```python
from build123d import *

# Parameters (mm, degrees)
SKETCH1_W           = 190
SKETCH1_H           = 219
BOSS_EXTRUDE1_DEPTH = 2
SKETCH4_W           = 70
SKETCH4_H           = 60
CUT_EXTRUDE1_DEPTH  = 4
SKETCH2_W           = 30
SKETCH2_H           = 2
BOSS_EXTRUDE2_DEPTH = 20
SKETCH3_W           = 190
SKETCH3_H           = 70
BOSS_EXTRUDE3_DEPTH = 72
SKETCH7_R           = 3
SKETCH7_R_2         = 4.5
BOSS_EXTRUDE4_DEPTH = 4
SKETCH8_R           = 3.5
CUT_EXTRUDE3_DEPTH  = 4
SKETCH9_R           = 2
BOSS_EXTRUDE5_DEPTH = 2
SKETCH10_R          = 0.95
CUT_EXTRUDE4_DEPTH  = 2
SKETCH11_R          = 1.875
SKETCH11_R_2        = 4.75
CUT_EXTRUDE5_DEPTH  = 4
SKETCH12_R          = 4.5
BOSS_EXTRUDE6_DEPTH = 72
SKETCH13_R          = 3.5
CUT_EXTRUDE6_DEPTH  = 4.5
FILLET1_START       = 2
FILLET1_DEPTH       = 73
FILLET1_START_2     = 22
FILLET1_2_DEPTH     = 53
FILLET1_START_3     = -1
FILLET1_3_DEPTH     = 23
SKETCH14_W          = 18
SKETCH14_H          = 15
CUT_EXTRUDE7_DEPTH  = 5
SKETCH15_R          = 2.1
BOSS_EXTRUDE7_DEPTH = 5.5


with BuildPart() as part:
    # Sketch1 → Boss-Extrude1 (new body)
    with BuildSketch(Plane(origin=(0, 0, 0), x_dir=(1, 0, 0), z_dir=(0, 1, 0))):
        with Locations((95, 109.5)):
            Rectangle(SKETCH1_W, SKETCH1_H)
    extrude(amount=BOSS_EXTRUDE1_DEPTH)

    # Sketch4 → Cut-Extrude1 (cut)
    with BuildSketch(Plane(origin=(0, 0, 0), x_dir=(1, 0, 0), z_dir=(0, 1, 0))):
        with Locations((54, 111)):
            Rectangle(SKETCH4_W, SKETCH4_H)
        with Locations((136, 111)):
            Rectangle(SKETCH4_W, SKETCH4_H)
        with Locations((136, 39)):
            Rectangle(SKETCH4_W, SKETCH4_H)
        with Locations((54, 39)):
            Rectangle(SKETCH4_W, SKETCH4_H)
    extrude(amount=CUT_EXTRUDE1_DEPTH, mode=Mode.SUBTRACT)

    # Sketch2 → Boss-Extrude2 (add)
    with BuildSketch(Plane(origin=(0, 2, 0), x_dir=(1, 0, 0), z_dir=(0, 1, 0))):
        with Locations((95, 1)):
            Rectangle(SKETCH2_W, SKETCH2_H)
        Polygon((160, 0), (190, 0), (190, 30), (188, 30), (188, 2), (160, 2), align=None)
        Polygon((190, 121), (190, 151), (156, 151), (156, 149), (188, 149), (188, 121), align=None)
    extrude(amount=BOSS_EXTRUDE2_DEPTH)

    # Sketch3 → Boss-Extrude3 (add)
    with BuildSketch(Plane(origin=(0, 2, 0), x_dir=(1, 0, 0), z_dir=(0, 1, 0))):
        with Locations((95, 184)):
            Rectangle(SKETCH3_W, SKETCH3_H)
        Polygon((188, 217), (120, 217), (120, 211), (117, 211), (117, 217), (112.8, 217), (112.8, 211), (109.8, 211), (109.8, 217), (2, 217), (2, 151), (109.8, 151), (109.8, 157), (112.8, 157), (112.8, 151), (117, 151), (117, 157), (120, 157), (120, 151), (188, 151), align=None, mode=Mode.SUBTRACT)
    extrude(amount=BOSS_EXTRUDE3_DEPTH)

    # Sketch7 → Boss-Extrude4 (add)
    with BuildSketch(Plane(origin=(0, 2, 0), x_dir=(1, 0, 0), z_dir=(0, 1, 0))):
        with Locations(Location((24, 208, 0), (0, 0, 90))):
            Circle(SKETCH7_R)
        with Locations(Location((24, 160, 0), (0, 0, 90))):
            Circle(SKETCH7_R)
        with Locations(Location((76, 193.5, 0), (0, 0, 90))):
            Circle(SKETCH7_R_2)
        with Locations(Location((76, 165.5, 0), (0, 0, 90))):
            Circle(SKETCH7_R_2)
    extrude(amount=BOSS_EXTRUDE4_DEPTH)

    # Sketch8 → Cut-Extrude3 (cut)
    with BuildSketch(Plane(origin=(0, 6, 0), x_dir=(1, 0, 0), z_dir=(0, 1, 0))):
        with Locations(Location((76, 193.5, 0), (0, 0, 270))):
            Circle(SKETCH8_R)
        with Locations(Location((76, 165.5, 0), (0, 0, 270))):
            Circle(SKETCH8_R)
    extrude(amount=-CUT_EXTRUDE3_DEPTH, mode=Mode.SUBTRACT)

    # Sketch9 → Boss-Extrude5 (add)
    with BuildSketch(Plane.ZY.offset(-188)):
        with Locations((-204.5, 55.5)):
            Circle(SKETCH9_R)
        with Locations((-163.5, 55.5)):
            Circle(SKETCH9_R)
        with Locations((-204.5, 27)):
            Circle(SKETCH9_R)
        with Locations((-163.5, 27)):
            Circle(SKETCH9_R)
    extrude(amount=BOSS_EXTRUDE5_DEPTH)

    # Sketch10 → Cut-Extrude4 (cut)
    with BuildSketch(Plane.ZY.offset(-186)):
        with Locations((-204.5, 55.5)):
            Circle(SKETCH10_R)
        with Locations((-163.5, 55.5)):
            Circle(SKETCH10_R)
        with Locations((-163.5, 27)):
            Circle(SKETCH10_R)
        with Locations((-204.5, 27)):
            Circle(SKETCH10_R)
    extrude(amount=-CUT_EXTRUDE4_DEPTH, mode=Mode.SUBTRACT)

    # Sketch11 → Cut-Extrude5 (cut)
    with BuildSketch(Plane.ZY.offset(-188)):
        with Locations((-196.5, 49.25)):
            Circle(SKETCH11_R)
        with Locations((-186.5, 49.25)):
            Circle(SKETCH11_R)
        with Locations((-176.5, 49.25)):
            Circle(SKETCH11_R)
        with Locations((-194.25, 35)):
            Circle(SKETCH11_R_2)
        with Locations((-179, 35)):
            Circle(SKETCH11_R_2)
    extrude(amount=-CUT_EXTRUDE5_DEPTH, mode=Mode.SUBTRACT)

    # Sketch12 → Boss-Extrude6 (add)
    with BuildSketch(Plane(origin=(0, 2, 0), x_dir=(1, 0, 0), z_dir=(0, 1, 0))):
        with Locations((5, 214)):
            Circle(SKETCH12_R)
        with Locations((5, 154)):
            Circle(SKETCH12_R)
        with Locations((185, 214)):
            Circle(SKETCH12_R)
        with Locations((185, 154)):
            Circle(SKETCH12_R)
    extrude(amount=BOSS_EXTRUDE6_DEPTH)

    # Sketch13 → Cut-Extrude6 (cut)
    with BuildSketch(Plane(origin=(0, 74, 0), x_dir=(1, 0, 0), z_dir=(0, 1, 0))):
        with Locations(Location((5, 214, 0), (0, 0, 270))):
            Circle(SKETCH13_R)
        with Locations(Location((5, 154, 0), (0, 0, 270))):
            Circle(SKETCH13_R)
        with Locations(Location((185, 214, 0), (0, 0, 270))):
            Circle(SKETCH13_R)
        with Locations(Location((185, 154, 0), (0, 0, 270))):
            Circle(SKETCH13_R)
    extrude(amount=-CUT_EXTRUDE6_DEPTH, mode=Mode.SUBTRACT)

    # Fillet1: read off the stored shape, not the designer's step
    # Fillet1 outline → Fillet1 (cut)
    with BuildSketch(Plane(origin=(0, 0, 0), x_dir=(1, 0, 0), z_dir=(0, 1, 0)).offset(FILLET1_START)):
        with BuildLine():
            Line((0, 149), (4.5, 149))
            ThreePointArc((4.5, 149), (1.318019485, 150.318019485), (0, 153.5))
            Line((0, 153.5), (0, 149))
        make_face()
        with BuildLine():
            ThreePointArc((188, 149.758342614), (186.80624304, 149.19375696), (185.5, 149))
            Line((185.5, 149), (188, 149))
            Line((188, 149), (188, 149.758342614))
        make_face()
        with BuildLine():
            Line((0, 219), (0, 214.5))
            ThreePointArc((0, 214.5), (1.318019485, 217.681980515), (4.5, 219))
            Line((4.5, 219), (0, 219))
        make_face()
        with BuildLine():
            Line((190, 219), (185.5, 219))
            ThreePointArc((185.5, 219), (188.681980515, 217.681980515), (190, 214.5))
            Line((190, 214.5), (190, 219))
        make_face()
    extrude(amount=FILLET1_DEPTH, mode=Mode.SUBTRACT)

    # Fillet1 2 outline → Fillet1 2 (cut)
    with BuildSketch(Plane(origin=(0, 0, 0), x_dir=(1, 0, 0), z_dir=(0, 1, 0)).offset(FILLET1_START_2)):
        with BuildLine():
            ThreePointArc((190, 153.5), (189.468626966, 151.378679657), (188, 149.758342614))
            Line((188, 149.758342614), (188, 149))
            Line((188, 149), (190, 149))
            Line((190, 149), (190, 153.5))
        make_face()
    extrude(amount=FILLET1_2_DEPTH, mode=Mode.SUBTRACT)

    # Fillet1 3 outline → Fillet1 3 (cut)
    with BuildSketch(Plane(origin=(0, 0, 0), x_dir=(1, 0, 0), z_dir=(0, 1, 0)).offset(FILLET1_START_3)):
        with BuildLine():
            Line((0, 219), (0, 214.5))
            ThreePointArc((0, 214.5), (1.318019485, 217.681980515), (4.5, 219))
            Line((4.5, 219), (0, 219))
        make_face()
        with BuildLine():
            Line((190, 219), (185.5, 219))
            ThreePointArc((185.5, 219), (188.681980515, 217.681980515), (190, 214.5))
            Line((190, 214.5), (190, 219))
        make_face()
    extrude(amount=FILLET1_3_DEPTH, mode=Mode.SUBTRACT)

    # Sketch14 → Cut-Extrude7 (cut)
    with BuildSketch(Plane.ZY):
        with Locations((-200, 19.5)):
            Rectangle(SKETCH14_W, SKETCH14_H)
    extrude(amount=-CUT_EXTRUDE7_DEPTH, mode=Mode.SUBTRACT)

    # Sketch15 → Boss-Extrude7 (add)
    with BuildSketch(Plane(origin=(0, 6, 0), x_dir=(1, 0, 0), z_dir=(0, 1, 0))):
        with Locations(Location((24, 208, 0), (0, 0, 270))):
            Circle(SKETCH15_R)
        with Locations(Location((24, 160, 0), (0, 0, 270))):
            Circle(SKETCH15_R)
    extrude(amount=BOSS_EXTRUDE7_DEPTH)


solid = part.part
```
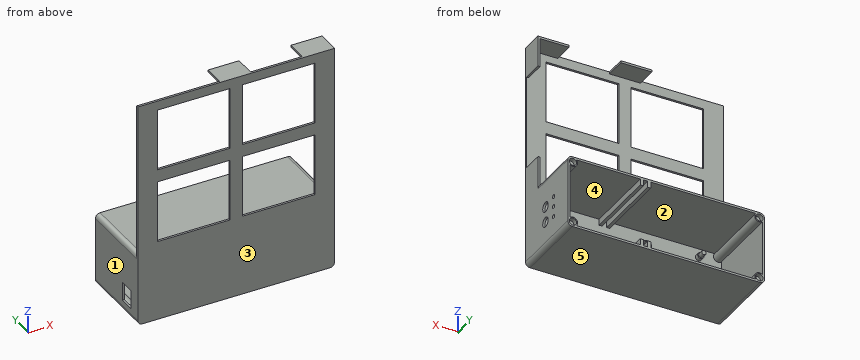
Can you work these out from the model? Positions are in its coordinate system, mm. Face numbers are marked on the shaded views. A direction names the side the tool comes from. Round coordinates to 2 decimals unless told otherwise and drop trailing zeros. Loops run counter-clockwise (first coordinate to the right, second up) from the corner with the lowest first, then second, coordinate; pieces in that order, holes last. Notation, with made-up numbers: M 41.5,-12 L 94.5,-12 A30 cw 94.5,17 Z; hole C 29,-21 d6. An arc over 180 degrees is marked long. Write item = value, one per line. Start each with the question number.
(1) I need wall thicknesses on line 1 along Z through (x, y) = (185, 71.7); line 2 along X through (y, z) = (73, -214); line 3 along Z through (x, y) = (93, 20). Which ranges of each line are inside material? Lowest first, please.
(2) Suppose I cut it at A-A on x = 130. Write out the boundary of the cut face in (y, z), plus the area to 3 significant figures.
(3) I'm going to push flat-ended pins straight in: P1, Ø1.3, axis at x = 24, z = -208, coming from the +Y side; P2, Ø3, axis at y = 12.5, z = -141, coming from the -X side; P3, Ø10, axis at x = 77.5, z = -163.5, coming from the +Y side. Where does each tip first touch, or does it pass through?
(4) Suppose I cut it at B-B on z = -22. Write out the boundary of the cut face in (x, y), plus the area to 3 significant figures.
(5) If we mould it in two halves opening along Z, with no side actions, what happens to the marked faces 3, 4 and 5? For each: released by +Z, released by -Z, zero draft, split by the parting line, or undercut.
(6) Suppose I cut it at D-D on z = -97.5. Write out the boundary of the cut face in (x, y).
(7) Which directions (+Z, -Z, +X, -X, +Y, -Y) give clear straight access to the entire face, cutting with the end or side of a thin tool? Please do the marked faces 1 and 2.
Answer block:
q1.line_1 = -219 to -217.5, -210.5 to -209.5, -158.5 to -157.5, -150.5 to -149
q1.line_2 = 0 to 1.5, 8.5 to 9.5, 109.8 to 112.8, 117 to 120, 180.5 to 181.5, 188.5 to 190
q1.line_3 = -219 to -217, -151 to -149, -2 to 0
q2.outline = M 0,-219 L 74,-219 L 74,-217 L 2,-217 L 2,-151 L 74,-151 L 74,-149 L 2,-149 L 2,-141 L 0,-141 Z; M 0,-81 L 2,-81 L 2,-69 L 0,-69 Z; M 0,-9 L 2,-9 L 2,0 L 0,0 Z
q2.area = 486 mm²
q3.P1 = 11.5
q3.P2 = 188
q3.P3 = 6
q4.outline = M 0,0 L 19,0 L 19,2 L 0,2 Z; M 89,0 L 101,0 L 101,2 L 89,2 Z; M 171,0 L 190,0 L 190,22 L 188,22 L 188,2 L 171,2 Z
q4.area = 140 mm²
q5.face_3 = zero draft
q5.face_4 = undercut
q5.face_5 = released by -Z
q6.outline = M 0,0 L 19,0 L 19,2 L 0,2 Z; M 89,0 L 101,0 L 101,2 L 89,2 Z; M 171,0 L 190,0 L 190,2 L 171,2 Z
q7.face_1 = +Z, -Z, -X, +Y, -Y
q7.face_2 = +Y
